For this review, take the finished solid that the model builds, in its own axes (mm). A direction names the side the tool comes from. Round coordinates to 2 decimals unless told otherwise and drop trailing zeros. Write each loop counter-clockwise with the first axis right and the second up, starting at its lowest first coordinate (ties: lowest second). Pieces come first, ordered by that corner, then holes. Notation, with made-up numbers: (-14.5, 3) - (-3.5, 3) arc R8 cw to (-3.5, 9) - close; hole circle Ø7 at (1.25, 63). An arc over 180 degrees is marked (long way). One line per item, written item: value. Start each with the question number.
Q1. For probe 1 along Y at (x, z) = (3.5, 7); probe 2 along Z at (x, y) = (8, 7.25); probe 3 along Z at (x, y) = (7.5, -7.5), list the stretches that pass through material, from the lowest coordinate up.
Q2. Clearance check with flat-ended pins moving along their axes: pin 1 Ø4 at (x, z) = (4, 3.5) entering from -Y; pin 2 Ø2 at (x, z) = (6.5, 6.5) entering from +Y; pin 3 Ø2 at (x, z) = (5.5, 2.5) entering from +Y. State where each tip first meets the part, or that it passes through.
Q3. Tool access review of faces 1 (the face through (4.93, 4.175, -4.65)), 2 (the face through (0, 4, 0)): name each direction out of +Z, -Z, +X, -X, +Y, -Y from which nothing blocks a thin tool from reaching the whole face with its end or side.
Q4. Add section A-A on z = 1. Write out the cut boundary in (x, y).
Q5. Add section B-B on z = -6.75. Write out the cut boundary in (x, y), and give its area (3 significant figures).
Q6. Mouldability with a two-part tool opening along Z and no side actions: class faces 3 (the face through (10, 0, -4)), 4 (the face through (5, -2.05, 0)) as +Z half, -Z half, draft (parallel to the pull), parting line (faces both ways), or undercut.
```python
from build123d import *

# Parameters (mm, degrees)
BASPROSKE_W         = 10
BASPROSKE_H         = 8.5
TOOTHCUT_DEPTH      = 16.636495771
TEETHCUTS_COUNT     = 15
TEETHCUTS_ANGLE     = 336
BORSKE_R            = 2.5
BORE_DEPTH          = 50.0000508
BOSS_EXTRUDE1_DEPTH = 10
CUT_EXTRUDE1_DEPTH  = 10


with BuildPart() as part:
    # BasProSke → Base-Revolve (revolve)
    with BuildSketch(Plane(origin=(0, 0, 0), x_dir=(1, 0, 0), z_dir=(0, 1, 0)), mode=Mode.PRIVATE) as base_revolve_sk:
        with Locations((5, 4.25)):
            Rectangle(BASPROSKE_W, BASPROSKE_H)
    revolve(base_revolve_sk.sketch.rotate(Axis((-10, 0, 0), (1, 0, 0)), 180), axis=Axis((-10, 0, 0), (1, 0, 0)))

    # TooCutSke → ToothCut (cut, through all)
    with BuildSketch(Plane(origin=(0, 0, 0), x_dir=(0, 0, -1), z_dir=(1, 0, 0))):
        with BuildLine():
            ThreePointArc((0.619547138, 6.21821215), (0, 6.249), (-0.619547138, 6.21821215))
            ThreePointArc((-0.619547138, 6.21821215), (-0.827197364, 7.394441061), (-1.477319646, 8.396426134))
            ThreePointArc((-1.477319646, 8.396426134), (0, 8.5254), (1.477319646, 8.396426134))
            ThreePointArc((1.477319646, 8.396426134), (0.827197364, 7.394441061), (0.619547138, 6.21821215))
        make_face()
    toothcut = extrude(amount=TOOTHCUT_DEPTH, mode=Mode.SUBTRACT)

    # TeethCuts: ToothCut ×15 about axis
    teethcuts_axis = Axis((-10, 0, 0), (1, 0, 0))
    for i in range(1, TEETHCUTS_COUNT):
        add(toothcut.rotate(teethcuts_axis, i * TEETHCUTS_ANGLE / (TEETHCUTS_COUNT - 1)), mode=Mode.SUBTRACT)

    # BorSke → Bore (cut, symmetric)
    with BuildSketch(Plane(origin=(0, 0, 0), x_dir=(0, 0, -1), z_dir=(1, 0, 0))):
        with Locations(Location((0, 0, 0), (0, 0, 180))):
            Circle(BORSKE_R)
    extrude(amount=BORE_DEPTH, both=True, mode=Mode.SUBTRACT)

    # Sketch1 → Boss-Extrude1 (add, through all)
    with BuildSketch(Plane(origin=(10, 0, 0), x_dir=(0, 0, -1), z_dir=(1, 0, 0))):
        with BuildLine():
            ThreePointArc((1.907223112, 2.05), (0, 2.8), (-1.907223112, 2.05))
            Line((-1.907223112, 2.05), (1.907223112, 2.05))
        make_face()
        with BuildLine():
            Line((1.907223112, -2.05), (-1.907223112, -2.05))
            ThreePointArc((-1.907223112, -2.05), (0, -2.8), (1.907223112, -2.05))
        make_face()
    extrude(amount=-BOSS_EXTRUDE1_DEPTH)

    # Sketch1<3> → Cut-Extrude1 (cut)
    with BuildSketch(Plane(origin=(10, 0, 0), x_dir=(0, 0, -1), z_dir=(1, 0, 0))):
        with BuildLine():
            Line((1.907223112, 2.05), (-1.907223112, 2.05))
            ThreePointArc((-1.907223112, 2.05), (-2.8, 0), (-1.907223112, -2.05))
            Line((-1.907223112, -2.05), (1.907223112, -2.05))
            ThreePointArc((1.907223112, -2.05), (2.567121415, -1.11798374), (2.8, 0))
            ThreePointArc((2.8, 0), (2.567121415, 1.11798374), (1.907223112, 2.05))
        make_face()
    extrude(amount=-CUT_EXTRUDE1_DEPTH, mode=Mode.SUBTRACT)


solid = part.part
```
Result set:
1. probe 1: y = -3 to -1.47, -0.04 to 1.5, 3.28 to 4.52
1. probe 2: z = -2.25 to -0.77, 0.77 to 2.25
1. probe 3: z = -3.76 to -2.7, -0.71 to 0.71, 2.7 to 3.76
2. pin 1: stops at y = -7.89
2. pin 2: stops at y = 4.52
2. pin 3: stops at y = 8.37
3. face 1: +X, -X
3. face 2: +Z, -Z, -X, +Y, -Y
4. outline: (0, -6.17) - (10, -6.17) - (10, -2.05) - (0, -2.05) - close; (0, 2.05) - (10, 2.05) - (10, 7.76) - (0, 7.76) - close
5. outline: (0, -2.97) - (10, -2.97) - (10, -1.38) - (0, -1.38) - close; (0, -0.06) - (10, -0.06) - (10, 1.48) - (0, 1.48) - close; (0, 3.05) - (10, 3.05) - (10, 4.5) - (0, 4.5) - close
5. area: 45.8 mm^2
6. face 3: draft
6. face 4: undercut
